from build123d import *

# Parameters (mm, degrees)
SKETCH1_W                                          = 10
SKETCH1_H                                          = 2.5
SKETCH2_R                                          = 4.5
BOSS_EXTRUDE1_DEPTH                                = 2.1
F_3_0_3_DIAMETER_HOLE1_D                           = 3
F_3_0_3_DIAMETER_HOLE1_DEPTH                       = 4.6
CBORE_FOR_M2_5_HEX_HEAD_MACHINE_SCREW1_D           = 3
CBORE_FOR_M2_5_HEX_HEAD_MACHINE_SCREW1_CBORE_D     = 6.126092487
CBORE_FOR_M2_5_HEX_HEAD_MACHINE_SCREW1_CBORE_DEPTH = 3


with BuildPart() as part:
    # Sketch1 → Revolve1 (revolve)
    with BuildSketch(Plane.XZ, mode=Mode.PRIVATE) as revolve1_sk:
        with Locations((5, 1.25)):
            Rectangle(SKETCH1_W, SKETCH1_H)
    revolve(revolve1_sk.sketch.rotate(Axis((0, 0, 2.5), (0, 0, -1)), 180), axis=Axis((0, 0, 2.5), (0, 0, -1)))

    # Sketch2 → Boss-Extrude1 (add)
    with BuildSketch(Plane.XY.offset(2.5)):
        Circle(SKETCH2_R)
    extrude(amount=BOSS_EXTRUDE1_DEPTH)

    # Ø3.0 (3) Diameter Hole1
    with Locations(Plane(origin=(0, 0, 0), x_dir=(-1, 0, 0), z_dir=(0, 0, -1))):
        with Locations((-4.75, -4.75), (4.75, -4.75), (4.75, 4.75), (-4.75, 4.75)):
            Hole(F_3_0_3_DIAMETER_HOLE1_D / 2, depth=F_3_0_3_DIAMETER_HOLE1_DEPTH)

    # CBORE for M2.5 Hex Head Machine Screw1 (through all)
    with Locations(Plane.XY.offset(4.6)):
        with Locations((0, 0)):
            CounterBoreHole(CBORE_FOR_M2_5_HEX_HEAD_MACHINE_SCREW1_D / 2, CBORE_FOR_M2_5_HEX_HEAD_MACHINE_SCREW1_CBORE_D / 2, CBORE_FOR_M2_5_HEX_HEAD_MACHINE_SCREW1_CBORE_DEPTH)


solid = part.part
Input: part model. Units: mm. Frame: model coordinates. A direction names the side the tool comes from. Give positions to 0.01 mm unless a question says otherwise; leave off trailing zeros. Write each loop counter-clockwise with the first axis right and the second up, starting at its lowest first coordinate (ties: lowest second). Pieces come first, ordered by that corner, then holes. Notation, with made-up numbers: M 24,50 L 68,50 A15 ccw 68,61 Z; hole C 0,-17 d3. An arc over 180 degrees is marked long. Write item = value, one per line. Start each with the question number.
1) First-contact query: pin 1 Ø4 at (x, y) = (1.5, 6.5) entering from +Z; pin 2 Ø1.8 at (x, y) = (-0.5, 1) entering from +Z. Flat tips, straight axial feed; report the tip coordinate or a pass-through.
2) Material intervals for line 1 along Y through (x, z) = (0, 0.6); line 2 along Y through (x, z) = (-4.75, 1.75); line 3 along Y through (x, z) = (-4.25, 0.55), sorted ascending. Write a range as [from, to].
3) Draft query along X for faces 1 (the flat face through (0, -2, 0)), 2 (the cylindrical face through (10, 0, 1)), 3 (the cylindrical face through (2.83, -1.17, 3.12)). Return one class per face: +X half, -X half, draft (parallel to the pull), parting line (faces both ways), or undercut.
4) Cut plane C-C on y = 4.75. Return the cut outline in (x, z), then the cut area to 3 significant figures.
5) Reachability of faces 4 (the flat face through (4.3, -2.1, 2.5)), 5 (the cylindrical face through (-5.86, -3.74, 1.27)) from +Z, -Z, +X, -X, +Y, -Y: full face, straight path, thin tool, end or side. Return the list, or none.
6) Cut plane A-A on y = 0. Return the cut outline in (x, z).
Solved:
q1.pin_1 = 2.5
q1.pin_2 = 1.6
q2.line_1 = [-10, -1.5], [1.5, 10]
q2.line_2 = [-8.8, -6.25], [-3.25, 3.25], [6.25, 8.8]
q2.line_3 = [-9.05, -6.16], [-3.34, 3.34], [6.16, 9.05]
q3.face_1 = draft
q3.face_2 = parting line
q3.face_3 = undercut
q4.outline = M -8.8,0 L -6.25,0 L -6.25,2.5 L -8.8,2.5 Z; M -3.25,0 L 3.25,0 L 3.25,2.5 L -3.25,2.5 Z; M 6.25,0 L 8.8,0 L 8.8,2.5 L 6.25,2.5 Z
q4.area = 29.0 mm2
q5.face_4 = +Z
q5.face_5 = +Z, -Z
q6.outline = M -10,0 L -1.5,0 L -1.5,1.6 L -3.06,1.6 L -3.06,4.6 L -4.5,4.6 L -4.5,2.5 L -10,2.5 Z; M 1.5,0 L 10,0 L 10,2.5 L 4.5,2.5 L 4.5,4.6 L 3.06,4.6 L 3.06,1.6 L 1.5,1.6 Z
